```python
from build123d import *

# Parameters (mm, degrees)
BOSS_EXTRUDE1_DEPTH = 4.572
SKETCH3_W           = 115.1315452
SKETCH3_H           = 4.572
BOSS_EXTRUDE2_DEPTH = 17.78
FILLET1_R           = 2.54
SKETCH4_W           = 121.92
SKETCH4_H           = 19.304
BOSS_EXTRUDE4_DEPTH = 5.08
SKETCH5_W           = 12.7
SKETCH5_H           = 6.35
CUT_EXTRUDE1_DEPTH  = 5.08
SKETCH6_R           = 1.27
CUT_EXTRUDE2_DEPTH  = 6.35


with BuildPart() as part:
    # Sketch2 → Boss-Extrude1 (new body)
    with BuildSketch(Plane(origin=(0, 0, 0), x_dir=(-1, 0, 0), z_dir=(0, 0, -1))):
        with BuildLine():
            Line((-62.487415839, 48.848476089), (52.644129361, 48.848476089))
            Line((52.644129361, 48.848476089), (41.713156468, -49.932022311))
            ThreePointArc((41.713156468, -49.932022311), (40.052782988, -53.157778108), (36.663977171, -54.453284069))
            Line((36.663977171, -54.453284069), (-46.507263649, -54.453284069))
            ThreePointArc((-46.507263649, -54.453284069), (-49.896069466, -53.157778108), (-51.556442946, -49.932022311))
            Line((-51.556442946, -49.932022311), (-62.487415839, 48.848476089))
        make_face()
    extrude(amount=BOSS_EXTRUDE1_DEPTH)

    # Sketch3 → Boss-Extrude2 (add)
    with BuildSketch(Plane(origin=(0, 48.848476089, 0), x_dir=(1, 0, 0), z_dir=(0, 1, 0))):
        with Locations((4.921643239, 2.286)):
            Rectangle(SKETCH3_W, SKETCH3_H)
    extrude(amount=BOSS_EXTRUDE2_DEPTH)

    # Fillet1
    fillet1_edges = [part.edges().sort_by_distance(p)[0] for p in [
        (62.487415839, 48.848476089, -2.286),
        (-52.644129361, 48.848476089, -2.286),
    ]]
    fillet(fillet1_edges, radius=FILLET1_R)

    # Sketch4 → Boss-Extrude4 (add)
    with BuildSketch(Plane(origin=(0, 66.628476089, 0), x_dir=(1, 0, 0), z_dir=(0, 1, 0))):
        with Locations((4.921643239, 2.286)):
            Rectangle(SKETCH4_W, SKETCH4_H)
    extrude(amount=BOSS_EXTRUDE4_DEPTH)

    # Sketch5 → Cut-Extrude1 (cut)
    with BuildSketch(Plane(origin=(0, 0, -4.572), x_dir=(-1, 0, 0), z_dir=(0, 0, -1))):
        with Locations((-4.921643239, -38.578284069)):
            Rectangle(SKETCH5_W, SKETCH5_H)
    extrude(amount=-CUT_EXTRUDE1_DEPTH, mode=Mode.SUBTRACT)

    # Sketch6 → Cut-Extrude2 (cut)
    with BuildSketch(Plane(origin=(0, 0, -4.572), x_dir=(-1, 0, 0), z_dir=(0, 0, -1))):
        Polygon((-14.921643239, 43.768476089), (-14.921643239, 41.228476089), (-14.921643239, 36.228476089), (-19.921643239, 36.228476089), (-19.921643239, -28.771523911), (5.478356761, -28.771523911), (5.478356761, -23.691523911), (8.018356761, -23.691523911), (8.018356761, 43.768476089), align=None)
        with Locations((-17.421643239, 38.728476089)):
            Circle(SKETCH6_R)
        with Locations((7.978356761, -26.271523911)):
            Circle(SKETCH6_R)
    extrude(amount=-CUT_EXTRUDE2_DEPTH, mode=Mode.SUBTRACT)


solid = part.part
```
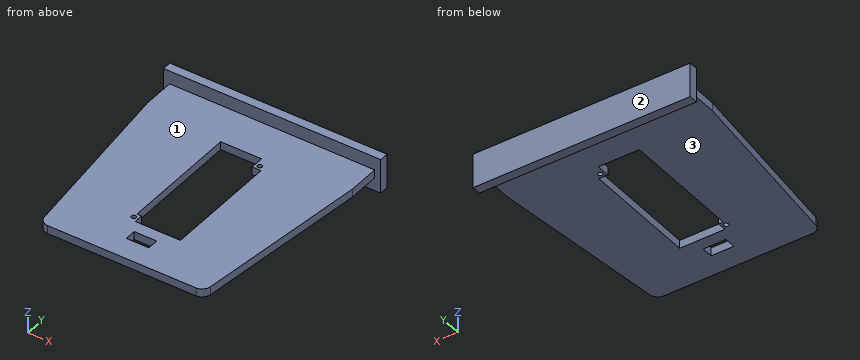
Input: part model. Units: mm. Frame: model coordinates. Face numbers are marked on the shaded views. A direction names the side the tool comes from. Give positions to 0.01 mm unless a question says otherwise; leave off trailing zeros. Order: outer loops, then holes, each group sorted by start corner. A loop starts at its lowest first (then second) coordinate and runs counter-clockwise, first axis right, second up. Notation, with made-up numbers: (59.5, 50) - (89.5, 50) arc R19 cw to (89.5, 83) - close; hole circle Ø9 at (30.25, 87). An arc over 180 degrees is marked (long way). One line per item, written item: value.
1. Cut plane D-D, the plane z = 4.5. Output: boundary loops of the cut face in (x, y), and give its area (3 significant figures).
Determined:
outline: (-56.04, 66.63) - (65.88, 66.63) - (65.88, 71.71) - (-56.04, 71.71) - close
area: 619 mm2
2. Cut plane A-A, the plane y = -38. Output: boundary loops of the cut face in (x, z).
Determined:
outline: (-43.03, -4.57) - (-1.43, -4.57) - (-1.43, 0) - (-43.03, 0) - close; (11.27, -4.57) - (52.88, -4.57) - (52.88, 0) - (11.27, 0) - close
3. Cut plane B-B, the plane x = -19. Output: boundary loops of the cut face in (y, z), and give its area (3 significant figures).
Determined:
outline: (-54.45, -4.57) - (66.63, -4.57) - (66.63, -11.94) - (71.71, -11.94) - (71.71, 7.37) - (66.63, 7.37) - (66.63, 0) - (-54.45, 0) - close
area: 652 mm2
4. Pin query (flat end, axial travel): pin 1 Ø3.5 at (x, y) = (-7.98, -26.27) entering from -Z; pin 2 Ø1.4 at (y, z) = (-37, -3) entering from -X; pin 3 Ø3 at (x, y) = (4, -34.5) entering from +Z. Return the tip coordinate at first contact, or that it passes through.
Determined:
pin 1: z = -4.57
pin 2: x = -43.22
pin 3: z = 0
5. Line query: probe 1 along Y at (x, z) = (7.5, -2.5); probe 2 along Y at (x, z) = (15.5, -1.75); probe 3 along X at (y, z) = (53, -1.75). Output: solid intervals per line, ascending.
Determined:
probe 1: -54.45 to -41.75, -35.4 to -28.77, 43.77 to 71.71
probe 2: -54.45 to -28.77, 36.23 to 71.71
probe 3: -52.64 to 62.49
6. Reachability of the marked faces 1, 2 and 3 from +Z, -Z, +X, -X, +Y, -Y: full face, straight path, thin tool, end or side. Return the list, or none.
Determined:
face 1: +Z, +X, -X, -Y
face 2: +Z, -Z, +X, -X, +Y
face 3: -Z, +X, -X, -Y
7. Cut plane C-C, the plane y = 17. Output: boundary loops of the cut face in (x, z), and give its area (3 significant figures).
Determined:
outline: (-49.12, -4.57) - (-8.02, -4.57) - (-8.02, 0) - (-49.12, 0) - close; (19.92, -4.57) - (58.96, -4.57) - (58.96, 0) - (19.92, 0) - close
area: 366 mm2
